from build123d import *

# Parameters (mm, degrees)
F0_R      = 50
F2_DEPTH  = 8
F4_R      = 2
F6_R      = 46
F7_DEPTH  = 2
F9_DEPTH  = 2
F8_R      = 1.5
F10_DEPTH = 2


with BuildPart() as f2:
    # F0 (on Top) → F2 (new body)
    with BuildSketch(Plane.XY):
        Circle(F0_R)
    extrude(amount=F2_DEPTH)

    # F4
    f4_edges = [f2.edges().sort_by_distance(p)[0] for p in [
        (-50, 0, 8),
    ]]
    fillet(f4_edges, radius=F4_R)

    # F6 (on face) → F7 (cut)
    with BuildSketch(Plane.XY.offset(8)):
        Circle(F6_R)
    extrude(amount=-F7_DEPTH, mode=Mode.SUBTRACT)

    # F8 (on face) → F9 (cut)
    with BuildSketch(Plane.XY.offset(6)):
        with BuildLine():
            ThreePointArc((-1.3134240992, -19.5237704918), (-1.0937541851, -18.9934404059), (-0.5634240992, -18.7737704918))
            Line((-0.5634240992, -18.7737704918), (0, -18.7737704918))
            Line((0, -18.7737704918), (0.5634240992, -18.7737704918))
            ThreePointArc((0.5634240992, -18.7737704918), (1.0937541851, -18.9934404059), (1.3134240992, -19.5237704918))
            Line((1.3134240992, -19.5237704918), (1.3134240992, -26.3196417335))
            ThreePointArc((1.3134240992, -26.3196417335), (2.4117736698, -28.9712921629), (5.0634240992, -30.0696417335))
            Line((5.0634240992, -30.0696417335), (7.2902552709, -30.0696417335))
            ThreePointArc((7.2902552709, -30.0696417335), (9.9419057003, -28.9712921629), (11.0402552709, -26.3196417335))
            Line((11.0402552709, -26.3196417335), (11.0402552709, -19.5237704918))
            ThreePointArc((11.0402552709, -19.5237704918), (11.259925185, -18.9934404059), (11.7902552709, -18.7737704918))
            Line((11.7902552709, -18.7737704918), (14.25, -18.7737704918))
            ThreePointArc((14.25, -18.7737704918), (16.9016504294, -17.6754209213), (18, -15.0237704918))
            Line((18, -15.0237704918), (18, 8.2737704918))
            ThreePointArc((18, 8.2737704918), (15.2027368941, 16.6809104679), (8.7900681537, 22.7950222666))
            Line((8.7900681537, 22.7950222666), (12.8468124166, 28.5337620023))
            ThreePointArc((12.8468124166, 28.5337620023), (12.9313132133, 28.9069994934), (12.7271455387, 29.2306693407))
            Line((12.7271455387, 29.2306693407), (11.0939971059, 30.3851502616))
            ThreePointArc((11.0939971059, 30.3851502616), (10.7207596148, 30.4696510582), (10.3970897675, 30.2654833836))
            Line((10.3970897675, 30.2654833836), (6.0233529733, 24.078320598))
            ThreePointArc((6.0233529733, 24.078320598), (3.0586137327, 24.8896799806), (0, 25.1944173204))
            ThreePointArc((0, 25.1944173204), (-3.0586137327, 24.8896799806), (-6.0233529733, 24.078320598))
            Line((-6.0233529733, 24.078320598), (-10.3970897675, 30.2654833836))
            ThreePointArc((-10.3970897675, 30.2654833836), (-10.7207596148, 30.4696510582), (-11.0939971059, 30.3851502616))
            Line((-11.0939971059, 30.3851502616), (-12.7271455387, 29.2306693407))
            ThreePointArc((-12.7271455387, 29.2306693407), (-12.9313132133, 28.9069994934), (-12.8468124166, 28.5337620023))
            Line((-12.8468124166, 28.5337620023), (-8.7900681537, 22.7950222666))
            ThreePointArc((-8.7900681537, 22.7950222666), (-15.2027368941, 16.6809104679), (-18, 8.2737704918))
            Line((-18, 8.2737704918), (-18, -15.0237704918))
            ThreePointArc((-18, -15.0237704918), (-16.9016504294, -17.6754209213), (-14.25, -18.7737704918))
            Line((-14.25, -18.7737704918), (-11.7902552709, -18.7737704918))
            ThreePointArc((-11.7902552709, -18.7737704918), (-11.259925185, -18.9934404059), (-11.0402552709, -19.5237704918))
            Line((-11.0402552709, -19.5237704918), (-11.0402552709, -26.3196417335))
            ThreePointArc((-11.0402552709, -26.3196417335), (-9.9419057003, -28.9712921629), (-7.2902552709, -30.0696417335))
            Line((-7.2902552709, -30.0696417335), (-5.0634240992, -30.0696417335))
            ThreePointArc((-5.0634240992, -30.0696417335), (-2.4117736698, -28.9712921629), (-1.3134240992, -26.3196417335))
            Line((-1.3134240992, -26.3196417335), (-1.3134240992, -19.5237704918))
        make_face()
        with BuildLine():
            Line((-14.25, 8.2737704918), (0, 8.2737704918))
            Line((0, 8.2737704918), (14.25, 8.2737704918))
            ThreePointArc((14.25, 8.2737704918), (14.7803300859, 8.0541005777), (15, 7.5237704918))
            Line((15, 7.5237704918), (15, -15.0237704918))
            ThreePointArc((15, -15.0237704918), (14.7803300859, -15.5541005777), (14.25, -15.7737704918))
            Line((14.25, -15.7737704918), (8.7902552709, -15.7737704918))
            ThreePointArc((8.7902552709, -15.7737704918), (8.259925185, -15.9934404059), (8.0402552709, -16.5237704918))
            Line((8.0402552709, -16.5237704918), (8.0402552709, -26.3196417335))
            ThreePointArc((8.0402552709, -26.3196417335), (7.8205853568, -26.8499718194), (7.2902552709, -27.0696417335))
            Line((7.2902552709, -27.0696417335), (5.0634240992, -27.0696417335))
            ThreePointArc((5.0634240992, -27.0696417335), (4.5330940133, -26.8499718194), (4.3134240992, -26.3196417335))
            Line((4.3134240992, -26.3196417335), (4.3134240992, -16.5237704918))
            ThreePointArc((4.3134240992, -16.5237704918), (4.0937541851, -15.9934404059), (3.5634240992, -15.7737704918))
            Line((3.5634240992, -15.7737704918), (0, -15.7737704918))
            Line((0, -15.7737704918), (-3.5634240992, -15.7737704918))
            ThreePointArc((-3.5634240992, -15.7737704918), (-4.0937541851, -15.9934404059), (-4.3134240992, -16.5237704918))
            Line((-4.3134240992, -16.5237704918), (-4.3134240992, -26.3196417335))
            ThreePointArc((-4.3134240992, -26.3196417335), (-4.5330940133, -26.8499718194), (-5.0634240992, -27.0696417335))
            Line((-5.0634240992, -27.0696417335), (-7.2902552709, -27.0696417335))
            ThreePointArc((-7.2902552709, -27.0696417335), (-7.8205853568, -26.8499718194), (-8.0402552709, -26.3196417335))
            Line((-8.0402552709, -26.3196417335), (-8.0402552709, -16.5237704918))
            ThreePointArc((-8.0402552709, -16.5237704918), (-8.259925185, -15.9934404059), (-8.7902552709, -15.7737704918))
            Line((-8.7902552709, -15.7737704918), (-14.25, -15.7737704918))
            ThreePointArc((-14.25, -15.7737704918), (-14.7803300859, -15.5541005777), (-15, -15.0237704918))
            Line((-15, -15.0237704918), (-15, 7.5237704918))
            ThreePointArc((-15, 7.5237704918), (-14.7803300859, 8.0541005777), (-14.25, 8.2737704918))
        make_face(mode=Mode.SUBTRACT)
        with BuildLine():
            Line((15, 9.7737704918), (0, 9.7737704918))
            Line((0, 9.7737704918), (-15, 9.7737704918))
            ThreePointArc((-15, 9.7737704918), (-9.6695107404, 18.6041395087), (0, 22.1944173204))
            ThreePointArc((0, 22.1944173204), (9.6695107404, 18.6041395087), (15, 9.7737704918))
        make_face(mode=Mode.SUBTRACT)
        with BuildLine():
            Line((-21, -8.3022542986), (-21, 4.2737704918))
            ThreePointArc((-21, 4.2737704918), (-25, 8.2737704918), (-29, 4.2737704918))
            Line((-29, 4.2737704918), (-29, -8.3022542986))
            ThreePointArc((-29, -8.3022542986), (-25, -12.3022542986), (-21, -8.3022542986))
        make_face()
        with BuildLine():
            Line((-26, -8.3022542986), (-26, 4.2737704918))
            ThreePointArc((-26, 4.2737704918), (-25, 5.2737704918), (-24, 4.2737704918))
            Line((-24, 4.2737704918), (-24, -8.3022542986))
            ThreePointArc((-24, -8.3022542986), (-25, -9.3022542986), (-26, -8.3022542986))
        make_face(mode=Mode.SUBTRACT)
        with BuildLine():
            ThreePointArc((21, -8.3022542986), (25, -12.3022542986), (29, -8.3022542986))
            Line((29, -8.3022542986), (29, 4.2737704918))
            ThreePointArc((29, 4.2737704918), (25, 8.2737704918), (21, 4.2737704918))
            Line((21, 4.2737704918), (21, -8.3022542986))
        make_face()
        with BuildLine():
            Line((26, 4.2737704918), (26, -8.3022542986))
            ThreePointArc((26, -8.3022542986), (25, -9.3022542986), (24, -8.3022542986))
            Line((24, -8.3022542986), (24, 4.2737704918))
            ThreePointArc((24, 4.2737704918), (25, 5.2737704918), (26, 4.2737704918))
        make_face(mode=Mode.SUBTRACT)
    extrude(amount=-F9_DEPTH, mode=Mode.SUBTRACT)

    # F8 (on face) → F10 (cut)
    with BuildSketch(Plane.XY.offset(6)):
        with Locations((-7.5, 16.0260769339)):
            Circle(F8_R)
        with Locations((7.5, 16.0260769339)):
            Circle(F8_R)
    extrude(amount=-F10_DEPTH, mode=Mode.SUBTRACT)


solid = f2.part
Verification items for the finished model (mm, model axes). Coordinates: 2 decimals unless noted, no trailing zeros. Order: outer loops, then holes, each group sorted by start corner. A loop starts at its lowest first (then second) coordinate and runs counter-clockwise, first axis right, second up. Notation, with made-up numbers: M 82,78 L 114,78 A25 ccw 114,116 Z; hole C 62.5,68.5 d5. An arc over 180 degrees is marked long. One line per item, written item: value. Start each with the question number.
Item 1: Thickness scan on probe 1 along Y at (x, z) = (-7.5, 4.55); probe 2 along X at (y, z) = (28, 5.75); probe 3 along Y at (x, z) = (20, 6.5). Record the ranges inside material, lowest first.
Item 2: Sectioned sample at B-B on z = 1.75. Record the cut outline in (x, y).
Item 3: Mould release check, pull along X, two halves, no side actions. Record for faces 1 (the flat face through (-1, 1, 0)), 2 (the cylindrical face through (-2.44, -29, 5.01)): pulls with the +X half, pulls with the -X half, needs draft (parallel to the pull), parting line crosses it, or undercut.
Item 4: Depth check by flat-ended pin: P1, Ø6, axis at x = 10.5, y = -1, coming from the -Z side; P2, Ø2, axis at y = -22, z = 5, coming from the -X side; P3, Ø1.5, axis at x = -30, y = 11.5, coming from the +Z side; P4, Ø0.6, axis at x = 6, z = 5.5, coming from the -Y side. Enter the tip coordinate at first touch or a pass-through.
Calculated:
1. probe 1: -49.43 to -30.06, -27.04 to 8.27, 9.77 to 14.53, 17.53 to 20.11, 26.17 to 49.43
1. probe 2: -41.42 to -12.47, -8.8 to 8.8, 12.47 to 41.42
1. probe 3: -45.76 to -41.42, 41.42 to 45.76
2. outline: C 0,0 d100
3. face 1: needs draft
3. face 2: undercut
4. P1: z = 0
4. P2: x = -45.38
4. P3: z = 6
4. P4: y = -49.67
